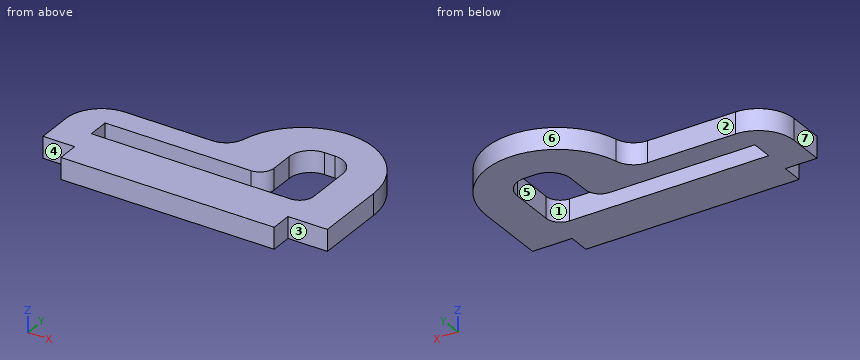
```python
from build123d import *

# Parameters (mm, degrees)
SALIENTE_EXTRUIR1_DEPTH = 3


with BuildPart() as part:
    # Croquis1 → Saliente-Extruir1 (new body)
    with BuildSketch(Plane.XY):
        with BuildLine():
            Line((-2.649110641, 0), (-15, 0))
            ThreePointArc((-15, 0), (-18.535533906, -1.464466094), (-20, -5))
            Line((-20, -5), (-20, -10))
            Line((-20, -10), (-15.546822742, -10))
            Line((-15.546822742, -10), (-15.546822742, -13))
            Line((-15.546822742, -13), (14.453177258, -13))
            Line((14.453177258, -13), (14.453177258, -10))
            Line((14.453177258, -10), (20, -10))
            Line((20, -10), (20, 0))
            ThreePointArc((20, 0), (11.161711866, 9.932292059), (0.269914892, 2.307692308))
            ThreePointArc((0.269914892, 2.307692308), (-0.788589622, 0.646606378), (-2.649110641, 0))
        make_face()
        with BuildLine():
            Line((-15.546822742, -6.391304348), (12.453177258, -6.391304348))
            ThreePointArc((12.453177258, -6.391304348), (13.86739082, -5.80551791), (14.453177258, -4.391304348))
            Line((14.453177258, -4.391304348), (14.453177258, -3.391304348))
            Line((14.453177258, -3.391304348), (14.453177258, 1.869565217))
            ThreePointArc((14.453177258, 1.869565217), (13.574497601, 3.990885561), (11.453177258, 4.869565217))
            Line((11.453177258, 4.869565217), (9.93812709, 4.869565217))
            ThreePointArc((9.93812709, 4.869565217), (7.816806747, 3.990885561), (6.93812709, 1.869565217))
            Line((6.93812709, 1.869565217), (6.93812709, -1.391304348))
            ThreePointArc((6.93812709, -1.391304348), (6.352340653, -2.80551791), (4.93812709, -3.391304348))
            Line((4.93812709, -3.391304348), (-15.546822742, -3.391304348))
            Line((-15.546822742, -3.391304348), (-15.546822742, -6.391304348))
        make_face(mode=Mode.SUBTRACT)
    extrude(amount=SALIENTE_EXTRUIR1_DEPTH)


solid = part.part
```
Design review of the part built by this model. Coordinates are the model's own, in mm. Face numbers are marked on the shaded views. A direction names the side the tool comes from. Round coordinates to 2 decimals unless told otherwise and drop trailing zeros. Write each loop counter-clockwise with the first axis right and the second up, starting at its lowest first coordinate (ties: lowest second). Pieces come first, ordered by that corner, then holes.
Item 1: We need section B-B on z = 1.45. Write out the cut boundary in (x, y).
Item 2: For the marked faces 1, 2, 3 and 4, list the 3-axis set-ups (+Z, -Z, +X, -X, +Y, -Y) from which the entire face can be reached by the end or side of a thin tool; tool diameter is ignored.
Item 3: We need section C-C on y = -2.5. Write out the cut boundary in (x, z).
Item 4: For probe 1 along Y at (x, z) = (-4.5, 2.55); probe 2 along X at (y, z) = (-5, 2.4); probe 3 along X at (y, z) = (4, 1.05), list the stretches that pass through material, from the lowest coordinate up.
Item 5: Clearance check with flat-ended pins moving along their axes: pin 1 Ø1.5 at (x, z) = (-17.5, 2) entering from -Y; pin 2 Ø1.5 at (y, z) = (-11.5, 1) entering from -X; pin 3 Ø0.9 at (y, z) = (-0.5, 2) entering from -X. State where each tip first meets the part, or that it passes through.
Item 6: We need section D-D on y = -11.25. Write out the cut boundary in (x, z), and give its area (3 significant figures).
Item 7: We need section A-A on x = -4. Write out the cut boundary in (y, z).
Item 8: The part is to be moulded in two halves that separate along Y. For the marked faces 5, 6 and 7, say which applies: +Y half, -Y half, draft (parallel to the pull), parting line (faces both ways), or undercut.
Returned:
1. outline: (-20, -10) - (-15.55, -10) - (-15.55, -13) - (14.45, -13) - (14.45, -10) - (20, -10) - (20, 0) arc R10 ccw to (0.27, 2.31) arc R3 cw to (-2.65, 0) - (-15, 0) arc R5 ccw to (-20, -5) - close; hole (-15.55, -6.39) - (12.45, -6.39) arc R2 ccw to (14.45, -4.39) - (14.45, 1.87) arc R3 ccw to (11.45, 4.87) - (9.94, 4.87) arc R3 ccw to (6.94, 1.87) - (6.94, -1.39) arc R2 cw to (4.94, -3.39) - (-15.55, -3.39) - close
2. face 1: +Z, -Z
2. face 2: +Z, -Z, -X, +Y
2. face 3: +Z, -Z, +X, -Y
2. face 4: +Z, -Z, -X, -Y
3. outline: (-19.33, 0) - (6.6, 0) - (6.6, 3) - (-19.33, 3) - close; (14.45, 0) - (20, 0) - (20, 3) - (14.45, 3) - close
4. probe 1: y = -13 to -6.39, -3.39 to 0
4. probe 2: x = -20 to -15.55, 14.36 to 20
4. probe 3: x = 0.83 to 7.83, 13.57 to 19.17
5. pin 1: stops at y = -10
5. pin 2: stops at x = -15.55
5. pin 3: stops at x = -17.93
6. outline: (-15.55, 0) - (14.45, 0) - (14.45, 3) - (-15.55, 3) - close
6. area: 90.0 mm2
7. outline: (-13, 0) - (-6.39, 0) - (-6.39, 3) - (-13, 3) - close; (-3.39, 0) - (0, 0) - (0, 3) - (-3.39, 3) - close
8. face 5: undercut
8. face 6: +Y half
8. face 7: draft
